Could you check a few things on this drawing? It's one solid part, dimensions in mm from its lowest x, y, z. A direction names the side the tool comes from. Round coordinates to 2 decimals unless told otherwise and drop trailing zeros. Write each loop counter-clockwise with the first axis right and the second up, starting at its lowest first coordinate (ties: lowest second). Pieces come first, ordered by that corner, then holes. Notation, with made-up numbers: (-2.75, 75) -> (47.25, 75) arc R17 ccw to (47.25, 95) -> close; hole circle Ø10 at (35.25, 62.5). An arc over 180 degrees is marked (long way). Return JSON: item names as keys, results as strings.
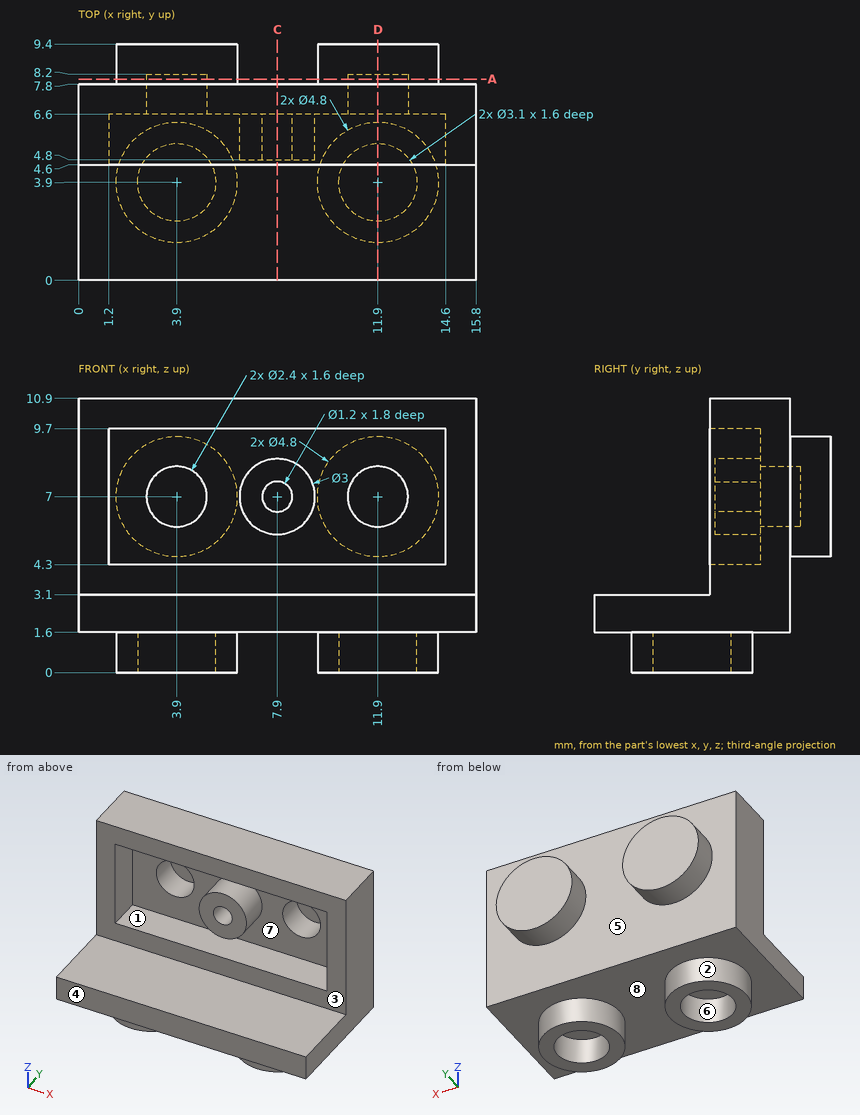
1) If I drill on probe 1 along X at (y, z) = (5.9, 7); probe 2 along Z at (x, y) = (11.5, 4.75); probe 3 along Y at (x, z) = (3.9, 0.4), over which ranges is the centre line in solid material (lowest first)? Write a range as [from, to].
Return value:
{"probe 1": "[0, 1.2], [6.4, 7.3], [8.5, 9.4], [14.6, 15.8]", "probe 2": "[1.6, 4.3], [9.7, 10.9]", "probe 3": "[1.5, 2.35], [5.45, 6.3]"}
2) I want a section at C-C, the plane x = 7.9. Please give me the cut outline in (y, z).
Return value:
{"outline": "(0, 1.6) -> (7.8, 1.6) -> (7.8, 10.9) -> (4.6, 10.9) -> (4.6, 9.7) -> (6.6, 9.7) -> (6.6, 8.5) -> (4.8, 8.5) -> (4.8, 7.6) -> (6.6, 7.6) -> (6.6, 6.4) -> (4.8, 6.4) -> (4.8, 5.5) -> (6.6, 5.5) -> (6.6, 4.3) -> (4.6, 4.3) -> (4.6, 3.1) -> (0, 3.1) -> close"}
3) For the marked faces 1, 2, 3, 4 and 5, which set-ups out of +Z, -Z, +X, -X, +Y, -Y let a thin tool reach every point of the face, with its end or its side?
Return value:
{"face 1": "-Y", "face 2": "-Z", "face 3": "+Z, +X, -X, -Y", "face 4": "+Z, -Z, +X, -X, -Y", "face 5": "+Y"}
4) I want a section at A-A, the plane y = 8. Please give me the cut outline in (x, z), and give its area (3 significant figures).
Return value:
{"outline": "circle Ø4.8 at (3.9, 7); circle Ø4.8 at (11.9, 7); hole circle Ø2.4 at (3.9, 7); hole circle Ø2.4 at (11.9, 7)", "area": "27.1 mm²"}
5) Will these pins go through, and if not, where does the flat tip stop? pin 1 Ø2.5 at (x, y) = (8.5, 3.5) entering from -Z; pin 2 Ø2.5 at (x, y) = (10.5, 2) entering from +Z; pin 3 Ø1.9 at (x, y) = (11.9, 3.9) entering from -Z; pin 4 Ø2.5 at (x, z) = (7, 7.5) entering from -Y.
Return value:
{"pin 1": "z = 0", "pin 2": "z = 3.1", "pin 3": "z = 1.6", "pin 4": "y = 4.8"}
6) Thinking about a two-plate mould opening in Y: for the marked faces 6, 7 and 8, which applies, pulls with the +Y half, pulls with the -Y half, needs draft (parallel to the pull), parting line crosses it, or undercut?
Return value:
{"face 6": "undercut", "face 7": "pulls with the -Y half", "face 8": "needs draft"}
7) I want a section at D-D, the plane x = 11.9. Please give me the cut outline in (y, z).
Return value:
{"outline": "(0, 1.6) -> (1.5, 1.6) -> (1.5, 0) -> (2.35, 0) -> (2.35, 1.6) -> (5.45, 1.6) -> (5.45, 0) -> (6.3, 0) -> (6.3, 1.6) -> (7.8, 1.6) -> (7.8, 4.6) -> (9.4, 4.6) -> (9.4, 9.4) -> (7.8, 9.4) -> (7.8, 10.9) -> (4.6, 10.9) -> (4.6, 9.7) -> (6.6, 9.7) -> (6.6, 8.2) -> (8.2, 8.2) -> (8.2, 5.8) -> (6.6, 5.8) -> (6.6, 4.3) -> (4.6, 4.3) -> (4.6, 3.1) -> (0, 3.1) -> close"}
